```python
from build123d import *

# Parameters (mm, degrees)
SKETCH3_R               = 73.025
BOSS_EXTRUDE2_DEPTH     = 25.4
CUT_EXTRUDE1_DEPTH      = 107.350652325
CUT_EXTRUDE1_DEPTH_BACK = 107.350652325
SKETCH4_R               = 3.96875
SKETCH4_R_2             = 12.7


with BuildPart() as part:
    # Sketch3 → Boss-Extrude2 (new body)
    with BuildSketch(Plane.XY):
        Circle(SKETCH3_R)
    extrude(amount=-BOSS_EXTRUDE2_DEPTH)

    # Sketch4 → Cut-Extrude1 (cut, two sides: drawn at the far end of the back side and taken through both)
    with BuildSketch(Plane.XY.offset(-CUT_EXTRUDE1_DEPTH_BACK)):
        with BuildLine():
            ThreePointArc((-39.686341225, -31.711737892), (-25.4, -43.994090512), (-7.62, -50.225248631))
            Line((-7.62, -50.225248631), (-7.62, -34.083591727))
            ThreePointArc((-7.62, -34.083591727), (-17.4625, -30.245937227), (-25.707256288, -23.64090944))
            Line((-25.707256288, -23.64090944), (-39.686341225, -31.711737892))
        make_face()
        with BuildLine():
            Line((7.62, -34.083591727), (7.62, -50.225248631))
            ThreePointArc((7.62, -50.225248631), (25.4, -43.994090512), (39.686341225, -31.711737892))
            Line((39.686341225, -31.711737892), (25.707256288, -23.64090944))
            ThreePointArc((25.707256288, -23.64090944), (17.4625, -30.245937227), (7.62, -34.083591727))
        make_face()
        with Locations((0, -25.4)):
            Circle(SKETCH4_R)
        with BuildLine():
            ThreePointArc((-47.306341225, 18.513510738), (-50.8, 0), (-47.306341225, -18.513510738))
            Line((-47.306341225, -18.513510738), (-33.327256288, -10.442682287))
            ThreePointArc((-33.327256288, -10.442682287), (-34.925, 0), (-33.327256288, 10.442682287))
            Line((-33.327256288, 10.442682287), (-47.306341225, 18.513510738))
        make_face()
        with BuildLine():
            Line((33.327256288, -10.442682287), (47.306341225, -18.513510738))
            ThreePointArc((47.306341225, -18.513510738), (50.8, 0), (47.306341225, 18.513510738))
            Line((47.306341225, 18.513510738), (33.327256288, 10.442682287))
            ThreePointArc((33.327256288, 10.442682287), (34.925, 0), (33.327256288, -10.442682287))
        make_face()
        Circle(SKETCH4_R_2)
        with Locations((-21.997045256, -12.7)):
            Circle(SKETCH4_R)
        with Locations((21.997045256, -12.7)):
            Circle(SKETCH4_R)
        with BuildLine():
            ThreePointArc((-7.62, 50.225248631), (-25.4, 43.994090512), (-39.686341225, 31.711737892))
            Line((-39.686341225, 31.711737892), (-25.707256288, 23.64090944))
            ThreePointArc((-25.707256288, 23.64090944), (-17.4625, 30.245937227), (-7.62, 34.083591727))
            Line((-7.62, 34.083591727), (-7.62, 50.225248631))
        make_face()
        with Locations((-21.997045256, 12.7)):
            Circle(SKETCH4_R)
        with Locations((21.997045256, 12.7)):
            Circle(SKETCH4_R)
        with BuildLine():
            Line((25.707256288, 23.64090944), (39.686341225, 31.711737892))
            ThreePointArc((39.686341225, 31.711737892), (25.4, 43.994090512), (7.62, 50.225248631))
            Line((7.62, 50.225248631), (7.62, 34.083591727))
            ThreePointArc((7.62, 34.083591727), (17.4625, 30.245937227), (25.707256288, 23.64090944))
        make_face()
        with Locations((0, 25.4)):
            Circle(SKETCH4_R)
    extrude(amount=CUT_EXTRUDE1_DEPTH + CUT_EXTRUDE1_DEPTH_BACK, mode=Mode.SUBTRACT)


solid = part.part
```
Source: CAD feature listing. Evaluate the final solid. Frame: model axes, mm. Coordinates: 2 decimals unless noted, no trailing zeros. Loops run counter-clockwise (first coordinate to the right, second up) from the corner with the lowest first, then second, coordinate; pieces in that order, holes last. Notation, with made-up numbers: M 0.5,20.5 L 38.5,20.5 A22 ccw 38.5,46.5 Z; hole C 15.5,-37.75 d4. An arc over 180 degrees is marked long. Put each result on its own line as item: value. Start each with the question number.
1) Cut plane B-B on z = -22.75. Give the number of separate pieces and of enclosed holes in the cut face, then the cut area to 3 significant figures.
2) Ray query, L1, parallel to Y at x = 0, z = -10.5 (3 decimals); L2, parallel to X at y = -14.5, z = -5.25; L3, parallel to X at y = -28, z = -5. Return the intervals inside material, ascending. Write a range as from..to.
3) Cut plane A-A on x = 0. Return the cut outline in (y, z) (3 decimals), then the cut area to 3 significant figures.
4) Pull-direction query (X, two-part tool) for faces 1 (the face through (-1, -15, -25.4)), 2 (the face through (25.63, 43.86, -12.88)); classes: pulls with the +X half, pulls with the -X half, needs draft (parallel to the pull), parting line crosses it, or undercut.
5) Cut plane C-C on y = 0. Return the cut outline in (x, z) (3 decimals), then the cut area to 3 significant figures.
6) Contact query for flat-ended pins moving along their axis: pin 1 Ø5 at (y, z) = (36.5, -7.5) entering from +X; pin 2 Ø8 at (y, z) = (-46, -11.5) entering from -X; pin 3 Ø10.5 at (x, y) = (0, -25.4) entering from +Z; pin 4 Ø8 at (y, z) = (45, -12.5) entering from +X. Output: stop coordinate, or through.
7) Cut plane D-D on y = -37. Return the cut outline in (x, z).
The answers:
1. separate pieces: 1
1. enclosed holes: 13
1. area: 13,100 mm²
2. L1: y = -73.025..-29.369, -21.431..-12.7, 12.7..21.431, 29.369..73.025
2. L2: x = -71.57..-48.69, -40.35..-25.53, -18.46..18.46, 25.53..40.35, 48.69..71.57
2. L3: x = -67.44..-33.26, -20.87..-3, 3..20.87, 33.26..67.44
3. outline: M -73.025,-25.4 L -29.369,-25.4 L -29.369,0 L -73.025,0 Z; M -21.431,-25.4 L -12.7,-25.4 L -12.7,0 L -21.431,0 Z; M 12.7,-25.4 L 21.431,-25.4 L 21.431,0 L 12.7,0 Z; M 29.369,-25.4 L 73.025,-25.4 L 73.025,0 L 29.369,0 Z
3. area: 2,660 mm²
4. face 1: needs draft
4. face 2: undercut
5. outline: M -73.025,-25.4 L -50.8,-25.4 L -50.8,0 L -73.025,0 Z; M -34.925,-25.4 L -12.7,-25.4 L -12.7,0 L -34.925,0 Z; M 12.7,-25.4 L 34.925,-25.4 L 34.925,0 L 12.7,0 Z; M 50.8,-25.4 L 73.025,-25.4 L 73.025,0 L 50.8,0 Z
5. area: 2,260 mm²
6. pin 1: stops at x = 64.63
6. pin 2: stops at x = -59.74
6. pin 3: stops at z = 0
6. pin 4: stops at x = 60.43
7. outline: M -62.96,-25.4 L -34.81,-25.4 L -34.81,0 L -62.96,0 Z; M -7.62,-25.4 L 7.62,-25.4 L 7.62,0 L -7.62,0 Z; M 34.81,-25.4 L 62.96,-25.4 L 62.96,0 L 34.81,0 Z
